```python
from build123d import *

# Parameters (mm, degrees)
SKETCH1_W           = 20
SKETCH1_H           = 35
SKETCH1_R           = 2.55
BOSS_EXTRUDE1_DEPTH = 10
CUT_EXTRUDE1_DEPTH  = 5
SKETCH3_R           = 2.55
CUT_EXTRUDE2_DEPTH  = 23.5
CUT_EXTRUDE4_START  = 10
CUT_EXTRUDE4_DEPTH  = 3
FILLET1_R           = 1


with BuildPart() as part:
    # Sketch1 → Boss-Extrude1 (new body)
    with BuildSketch(Plane.XY):
        Rectangle(SKETCH1_W, SKETCH1_H)
        with Locations((0, -10)):
            Circle(SKETCH1_R, mode=Mode.SUBTRACT)
        Circle(SKETCH1_R, mode=Mode.SUBTRACT)
    extrude(amount=BOSS_EXTRUDE1_DEPTH)

    # Sketch2 → Cut-Extrude1 (cut)
    with BuildSketch(Plane.XY):
        with BuildLine():
            Line((-5, 12.5), (-5, 17.5))
            Line((-5, 17.5), (10, 17.5))
            Line((10, 17.5), (10, 7.5))
            Line((10, 7.5), (0, 7.5))
            ThreePointArc((0, 7.5), (-3.535533906, 8.964466094), (-5, 12.5))
        make_face()
    extrude(amount=CUT_EXTRUDE1_DEPTH, mode=Mode.SUBTRACT)

    # Sketch3 → Cut-Extrude2 (cut, through all)
    with BuildSketch(Plane.XY):
        with Locations((0, 12.5)):
            Circle(SKETCH3_R)
    extrude(amount=CUT_EXTRUDE2_DEPTH, mode=Mode.SUBTRACT)

    # Sketch4 → Cut-Extrude4 (cut)
    with BuildSketch(Plane.XY.offset(CUT_EXTRUDE4_START)):
        with BuildLine():
            Line((-5, -10), (-5, 0))
            ThreePointArc((-5, 0), (0, 5), (5, 0))
            Line((5, 0), (5, -10))
            ThreePointArc((5, -10), (0, -15), (-5, -10))
        make_face()
    extrude(amount=-CUT_EXTRUDE4_DEPTH, mode=Mode.SUBTRACT)

    # Fillet1
    fillet1_edges = [part.edges().sort_by_distance(p)[0] for p in [
        (10, 7.5, 2.5),
        (-5, 17.5, 2.5),
        (-3.535533906, 8.964466094, 5),
        (5, 7.5, 5),
        (10, 12.5, 5),
        (2.5, 17.5, 5),
        (-5, 15, 5),
        (-5, -5, 10),
        (0, 5, 7),
        (5, -5, 10),
        (0, -15, 7),
        (-5, -5, 7),
        (5, -5, 7),
        (0, -15, 10),
        (0, 5, 10),
        (10, 17.5, 7.5),
        (10, -17.5, 5),
        (-10, -17.5, 5),
        (-10, 17.5, 5),
    ]]
    fillet(fillet1_edges, radius=FILLET1_R)


solid = part.part
```
The listing builds one solid part. Answer for the finished solid, in the listing's coordinates (mm). A direction names the side the tool comes from. Give positions to 0.01 mm unless a question says otherwise; leave off trailing zeros. Write each loop counter-clockwise with the first axis right and the second up, starting at its lowest first coordinate (ties: lowest second). Pieces come first, ordered by that corner, then holes. Notation, with made-up numbers: (-36, 67) - (-13, 67) arc R25 ccw to (-13, 94) - close; hole circle Ø9 at (14.25, 82.25). An arc over 180 degrees is marked (long way). Use one line per item in the form item = value. Start each with the question number.
1) Find section C-C on x = 6.75. Determine the outline of the cut face in (y, z), plus the area to 3 significant figures.
2) Find section B-B on y = 14. Determine the outline of the cut face in (x, z), plus the area to 3 significant figures.
3) A tool of negligible diameter and unlimited length cuts with its end or side. For faces 4 (the face through (-5.301, 17.215, 2.028)), 5 (the face through (-4.715, -4.93, 7.301)), 6 (the face through (-5, 4, 10)), from which of +Z, -Z, +X, -X, +Y, -Y can it reach the whole face along a straight path? Write none if from no direction.
4) Consider line 1 along Y through (x, z) = (0, 8.85); line 2 along Y through (x, z) = (0, 3); line 3 along X through (y, z) = (-10, 2). Determine where each line is inside the solid, lowest interval first. Write a range as from..to.
5) Find section D-D on z = 2.25. Determine the outline of the cut face in (x, y).
6) The mould has two halves that part along X. Classify faces 1 (the face through (5, 7.5, 2)), 2 (the face through (5, -4.9, 8.5)), 3 (the face through (9.699, -17.215, 5.07)): pulls with the +X half, pulls with the -X half, needs draft (parallel to the pull), parting line crosses it, or undercut.
7) Flat-ended cylindrical pins translate along their axes: pin 1 Ø3 at (x, z) = (6.5, 2.5) entering from +Y; pin 2 Ø4.5 at (y, z) = (15, 2.5) entering from +X; pin 3 Ø4.5 at (x, y) = (0, -10) entering from +Z; pin 4 Ø6.5 at (x, y) = (0, 12.5) entering from -Z. Find the tip coordinate at first contact, or state that the pin passes through.
8) Find section A-A on z = 8.5. Determine the outline of the cut face in (x, y), plus the area to 3 significant figures.
Geometry results:
q1.outline = (-17.5, 0) - (7.5, 0) - (7.5, 4) arc R1 cw to (8.5, 5) - (16.5, 5) arc R1 ccw to (17.5, 6) - (17.5, 10) - (-17.5, 10) - close
q1.area = 300 mm2
q2.outline = (-10, 0) - (-5, 0) - (-5, 4) arc R1 cw to (-4, 5) - (-2.06, 5) - (-2.06, 10) - (-10, 10) - close; (2.06, 5) - (9, 5) arc R1 ccw to (10, 6) - (10, 10) - (2.06, 10) - close
q2.area = 104 mm2
q3.face_4 = -Z, +X, +Y
q3.face_5 = +Z
q3.face_6 = +Z, +X, -X, +Y, -Y
q4.line_1 = -17.5..-15, 5..9.95, 15.05..17.5
q4.line_2 = -17.5..-12.55, -7.45..-2.55, 2.55..7.5
q4.line_3 = -10..-2.55, 2.55..10
q5.outline = (-10, -16.5) arc R1 ccw to (-9, -17.5) - (9, -17.5) arc R1 ccw to (10, -16.5) - (10, 6.5) arc R1 ccw to (9, 7.5) - (0, 7.5) arc R5 cw to (-5, 12.5) - (-5, 16.5) arc R1 ccw to (-6, 17.5) - (-9, 17.5) arc R1 ccw to (-10, 16.5) - close; hole circle Ø5.1 at (0, -10); hole circle Ø5.1 at (0, 0)
q6.face_1 = needs draft
q6.face_2 = undercut
q6.face_3 = pulls with the +X half
q7.pin_1 = 7.5
q7.pin_2 = -4.66
q7.pin_3 = through
q7.pin_4 = 5
q8.outline = (-10, -16.5) arc R1 ccw to (-9, -17.5) - (9, -17.5) arc R1 ccw to (10, -16.5) - (10, 16.5) arc R1 ccw to (9, 17.5) - (-9, 17.5) arc R1 ccw to (-10, 16.5) - close; hole (-5, -10) arc R5 ccw to (5, -10) - (5, 0) arc R5 ccw to (-5, 0) - close; hole circle Ø5.1 at (0, 12.5)
q8.area = 500 mm2
